```python
from build123d import *

# Parameters (mm, degrees)
SKETCH1_R           = 12.5
BOSS_EXTRUDE1_DEPTH = 17
SKETCH2_R           = 20
BOSS_EXTRUDE2_DEPTH = 25.425
SKETCH3_R           = 12.7
BOSS_EXTRUDE3_DEPTH = 31.75
SKETCH6_W           = 6.35
SKETCH6_H           = 3.175
BOSS_EXTRUDE6_DEPTH = 31.75
SKETCH4_R           = 20
BOSS_EXTRUDE4_DEPTH = 25.425
SKETCH5_R           = 12.5
BOSS_EXTRUDE5_DEPTH = 17


with BuildPart() as part:
    # Sketch1 → Boss-Extrude1 (new body)
    with BuildSketch(Plane.XY):
        Circle(SKETCH1_R)
    extrude(amount=-BOSS_EXTRUDE1_DEPTH)

    # Sketch2 → Boss-Extrude2 (add)
    with BuildSketch(Plane(origin=(0, 0, -17), x_dir=(-1, 0, 0), z_dir=(0, 0, -1))):
        with Locations(Location((0, 0, 0), (0, 0, 180))):
            Circle(SKETCH2_R)
    extrude(amount=BOSS_EXTRUDE2_DEPTH)

    # Sketch3 → Boss-Extrude3 (add)
    with BuildSketch(Plane(origin=(0, 0, -42.425), x_dir=(-1, 0, 0), z_dir=(0, 0, -1))):
        Circle(SKETCH3_R)
    extrude(amount=BOSS_EXTRUDE3_DEPTH)

    # Sketch6 → Boss-Extrude6 (add)
    with BuildSketch(Plane(origin=(0, 0, -74.175), x_dir=(-1, 0, 0), z_dir=(0, 0, -1))):
        with Locations((0, 13.884222124)):
            Rectangle(SKETCH6_W, SKETCH6_H)
    extrude(amount=-BOSS_EXTRUDE6_DEPTH)

    # Sketch4 → Boss-Extrude4 (add)
    with BuildSketch(Plane(origin=(0, 0, -74.175), x_dir=(-1, 0, 0), z_dir=(0, 0, -1))):
        with Locations(Location((0, 0, 0), (0, 0, 180))):
            Circle(SKETCH4_R)
    extrude(amount=BOSS_EXTRUDE4_DEPTH)

    # Sketch5 → Boss-Extrude5 (add)
    with BuildSketch(Plane(origin=(0, 0, -99.6), x_dir=(-1, 0, 0), z_dir=(0, 0, -1))):
        with Locations(Location((0, 0, 0), (0, 0, 180))):
            Circle(SKETCH5_R)
    extrude(amount=BOSS_EXTRUDE5_DEPTH)


solid = part.part
```
Geometry check sheet. Reference: the model listing, model coordinates, mm. A direction names the side the tool comes from. Round coordinates to 2 decimals unless told otherwise and drop trailing zeros. Loops run counter-clockwise (first coordinate to the right, second up) from the corner with the lowest first, then second, coordinate; pieces in that order, holes last. Notation, with made-up numbers: (78, 48) -> (117, 48) arc R12 cw to (117, 63) -> close; hole circle Ø3 at (41.5, 46). An arc over 180 degrees is marked (long way). Use a Markdown table: item, result.
(1) Scan lines: probe 1 along Z at (x, y) = (-6.5, 11) (3 decimals); probe 2 along Z at (x, y) = (-1.5, -12.5); probe 3 along Y at (x, z) = (0.5, -96.5). Record each from-to range of solid material in increasing order.
Calculated:
| item | result |
|---|---|
| probe 1 | -99.6 to -74.175, -42.425 to -17 |
| probe 2 | -99.6 to -17 |
| probe 3 | -19.99 to 19.99 |
(2) Sectioned sample at A-A (x = -17.5). Enter the section's corners in (y, z) (3 decimals).
Calculated:
| item | result |
|---|---|
| outline | (-9.682, -99.6) -> (9.682, -99.6) -> (9.682, -74.175) -> (-9.682, -74.175) -> close; (-9.682, -42.425) -> (9.682, -42.425) -> (9.682, -17) -> (-9.682, -17) -> close |
(3) Sectioned sample at D-D (z = -33). Enter the section's corners in (x, y), then the cut area to 3 significant figures.
Calculated:
| item | result |
|---|---|
| outline | circle Ø40 at (0, 0) |
| area | 1,260 mm² |
(4) Sectioned sample at B-B (y = 0). Enter the section's corners in (x, z) (3 decimals).
Calculated:
| item | result |
|---|---|
| outline | (-20, -99.6) -> (-12.5, -99.6) -> (-12.5, -116.6) -> (12.5, -116.6) -> (12.5, -99.6) -> (20, -99.6) -> (20, -74.175) -> (12.7, -74.175) -> (12.7, -42.425) -> (20, -42.425) -> (20, -17) -> (12.5, -17) -> (12.5, 0) -> (-12.5, 0) -> (-12.5, -17) -> (-20, -17) -> (-20, -42.425) -> (-12.7, -42.425) -> (-12.7, -74.175) -> (-20, -74.175) -> close |
(5) Sectioned sample at C-C (x = 0). Enter the section's corners in (y, z) (3 decimals).
Calculated:
| item | result |
|---|---|
| outline | (-20, -99.6) -> (-12.5, -99.6) -> (-12.5, -116.6) -> (12.5, -116.6) -> (12.5, -99.6) -> (20, -99.6) -> (20, -74.175) -> (15.472, -74.175) -> (15.472, -42.425) -> (20, -42.425) -> (20, -17) -> (12.5, -17) -> (12.5, 0) -> (-12.5, 0) -> (-12.5, -17) -> (-20, -17) -> (-20, -42.425) -> (-12.7, -42.425) -> (-12.7, -74.175) -> (-20, -74.175) -> close |
(6) Go/stop test with flat-tipped pins: P1, Ø6, axis at x = 11, z = -88, coming from the +Y side; P2, Ø2, axis at x = 15, z = -52.5, coming from the -Y side; P3, Ø1, axis at y = 14.5, z = -56.5, coming from the -X side (3 decimals); P4, Ø3.5, axis at y = 14.5, z = -57.5, coming from the +X side (3 decimals). Record where each tip stops, or that it passes through.
Calculated:
| item | result |
|---|---|
| P1 | y = 18.33 |
| P2 | through |
| P3 | x = -3.175 |
| P4 | x = 3.175 |
(7) Mould release check, pull along Z, two halves, no side actions. Record for faces 6 (the cylindrical face through (11.923, -3.755, -107.981)), 7 (the flat face through (0, 0, 0)), 8 (the flat face through (13, 0, -42.425)): released by +Z, released by -Z, zero draft, split by the parting line, or undercut.
Calculated:
| item | result |
|---|---|
| face 6 | zero draft |
| face 7 | released by +Z |
| face 8 | undercut |
(8) Set-up check for faces 1 (the flat face through (9, -9, -17)), 2 (the cylindrical face through (0.51, -12.69, -58.08)), 3 (the flat face through (0, 15.472, -59)), 4 (the flat face through (9, -9, -99.6)), 5 (the flat face through (3.175, 14, -59)): record each of +Z, -Z, +X, -X, +Y, -Y from which the full face is reachable in a straight line by a thin tool's end or side.
Calculated:
| item | result |
|---|---|
| face 1 | +Z |
| face 2 | none |
| face 3 | +X, -X, +Y |
| face 4 | -Z |
| face 5 | +X, +Y |
